Geometry: final body of the model. Coordinates: model frame, mm. Coordinates: 2 decimals unless noted, no trailing zeros. Loops run counter-clockwise (first coordinate to the right, second up) from the corner with the lowest first, then second, coordinate; pieces in that order, holes last. Notation, with made-up numbers: (87, -27.5) - (117, -27.5) arc R15 cw to (117, -17.5) - close; hole circle Ø8 at (4.5, -14). An arc over 180 degrees is marked (long way). Put each result on its own line as item: value. Start each with the question number.
1) Section A-A on y = 0. Output: boundary loops of the cut face in (x, z).
2) Section B-B on z = 0. Output: boundary loops of the cut face in (x, y).
3) Draft query along Y for faces 1 (the flat face through (-6.35, 3, -3)), 2 (the cylindrical face through (-1.388, 0.061, -5.052)), 3 (the cylindrical face through (0.089, -2.432, -5.866)). Return one class per face: +Y half, -Y half, draft (parallel to the pull), parting line (faces both ways), or undercut.
4) Contact query for flat-ended pins moving along their axis: pin 1 Ø6 at (x, z) = (-4, -3) entering from -Y; pin 2 Ø6 at (x, z) = (-1, -4.5) entering from +Y; pin 3 Ø3 at (x, y) = (0, 2) entering from -Z. Output: stop coordinate, or through.
5) Section D-D on x = 4.75. Output: boundary loops of the cut face in (y, z).
6) Section C-C on x = 0.25. Output: boundary loops of the cut face in (y, z).
7) Material intervals for line 1 along X through (y, z) = (0, -4.85); line 2 along Y through (x, z) = (3.25, 0), sorted ascending. Write a range as from..to.
```python
from build123d import *

# Parameters (mm, degrees)
SKETCH1_R           = 6.35
SKETCH1_R_2         = 3.96875
EXTRUDE1_DEPTH      = 6.35
EXTRUDE1_DEPTH_BACK = 6.35
CUT_EXTRUDE1_START  = -6.35
SKETCH2_R           = 1.3890625
CUT_EXTRUDE1_DEPTH  = 12.7


with BuildPart() as part:
    # Sketch1 → Extrude1 (new body, two sides)
    with BuildSketch(Plane(origin=(0, 0, 0), x_dir=(0, 0, -1), z_dir=(1, 0, 0))) as extrude1_sk:
        Circle(SKETCH1_R)
        Circle(SKETCH1_R_2, mode=Mode.SUBTRACT)
    extrude(amount=EXTRUDE1_DEPTH)
    extrude(extrude1_sk.sketch, amount=-EXTRUDE1_DEPTH_BACK)

    # Sketch2 → Cut-Extrude1 (cut)
    with BuildSketch(Plane.XY.offset(CUT_EXTRUDE1_START)):
        Circle(SKETCH2_R)
    extrude(amount=CUT_EXTRUDE1_DEPTH, mode=Mode.SUBTRACT)


solid = part.part
```
Answer block:
1. outline: (-6.35, -6.35) - (-1.39, -6.35) - (-1.39, -3.97) - (-6.35, -3.97) - close; (-6.35, 3.97) - (-1.39, 3.97) - (-1.39, 6.35) - (-6.35, 6.35) - close; (1.39, -6.35) - (6.35, -6.35) - (6.35, -3.97) - (1.39, -3.97) - close; (1.39, 3.97) - (6.35, 3.97) - (6.35, 6.35) - (1.39, 6.35) - close
2. outline: (-6.35, -6.35) - (6.35, -6.35) - (6.35, -3.97) - (-6.35, -3.97) - close; (-6.35, 3.97) - (6.35, 3.97) - (6.35, 6.35) - (-6.35, 6.35) - close
3. face 1: draft
3. face 2: undercut
3. face 3: parting line
4. pin 1: stops at y = -6.35
4. pin 2: stops at y = 6.17
4. pin 3: stops at z = -6.28
5. outline: circle Ø12.7 at (0, 0); hole circle Ø7.94 at (0, 0)
6. outline: (-1.37, -6.2) - (-1.37, -3.73) arc R3.97 cw to (-1.37, 3.73) - (-1.37, 6.2) arc R6.35 ccw to start; (1.37, -6.2) arc R6.35 ccw to (1.37, 6.2) - (1.37, 3.73) arc R3.97 cw to (1.37, -3.73) - close
7. line 1: x = -6.35..-1.39, 1.39..6.35
7. line 2: y = -6.35..-3.97, 3.97..6.35
